Source: three-view drawing plus pictorial views. Frame: mm from the lowest corner of the part. A direction names the side the tool comes from. Coordinates: 2 decimals unless noted, no trailing zeros. Write each loop counter-clockwise with the first axis right and the second up, starting at its lowest first coordinate (ties: lowest second). Pieces come first, ordered by that corner, then holes. Notation, with made-up numbers: (40.25, -10) -> (91.25, -10) arc R22 cw to (91.25, 9) -> close; hole circle Ø4 at (10.25, 17). An arc over 180 degrees is marked (long way). One line per item, written item: value. Start each with the question number.
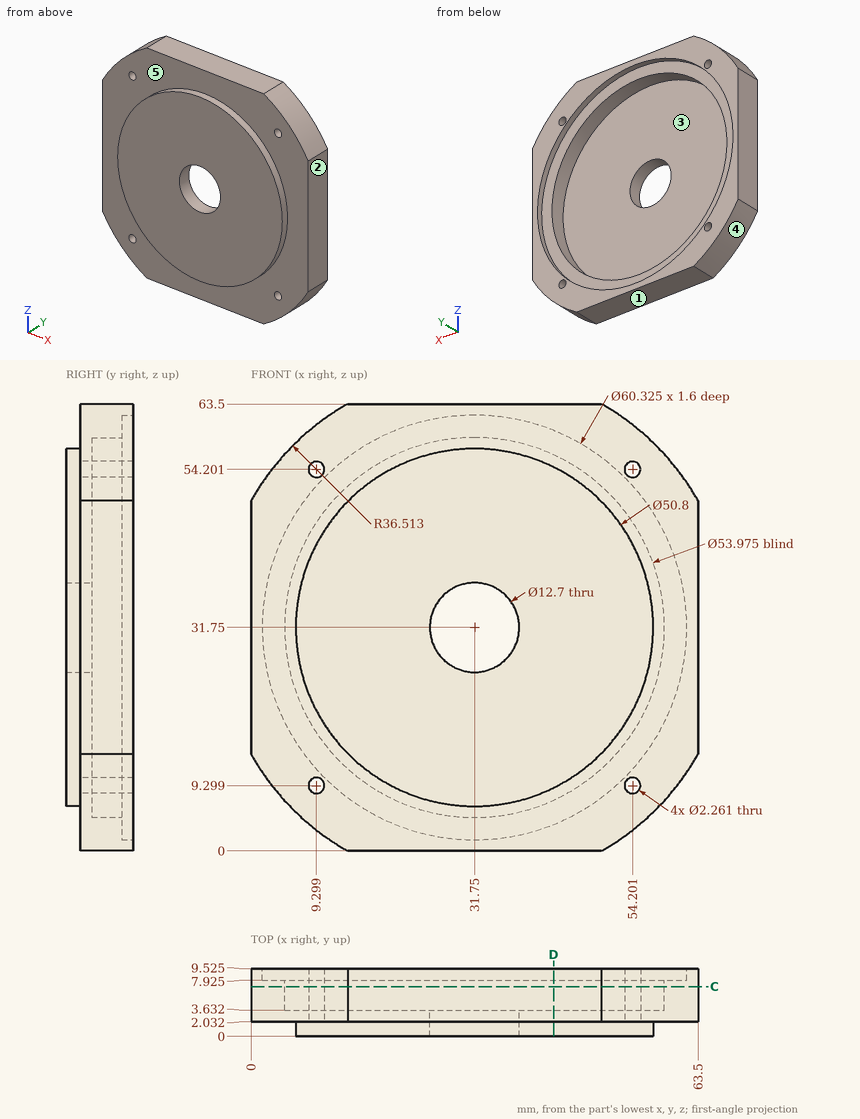
Q1. Draft query along Z for the marked faces 1, 2 and 3. Return one class per face: pulls with the +Z half, pulls with the -Z half, needs draft (parallel to the pull), parting line crosses it, or undercut.
Q2. First-contact query: P1, Ø12, axis at x = 47, z = 28.5, coming from the +Y side; P2, Ø5, axis at y = 1.5, z = 26.5, coming from the -X side; P3, Ø1.5, axis at x = 33.5, y = 1, coming from the +Z side. Flat tips, straight axial feed; report the tip coordinate or a pass-through.
Q3. Cut plane C-C on y = 7. Count the separate pieces of the cut face and the enclosed holes in it, and give its area (3 significant figures).
Q4. Access query for the marked faces 4 and 5. Directions: +Z, -Z, +X, -X, +Y, -Y. A direction counts if a zero-diameter tool reaches every point of the face in a straight line with its end or side. Return the directions, or none.
Q5. Line query: L1, parallel to Z at x = 31.75, y = 8.6; L2, parallel to X at y = 3, z = 54.5; L3, parallel to Y at x = 40.5, z = 27. Output: solid intervals per line, ascending. Write a range as from..to.
Q6. Cut plane D-D on x = 43. Output: boundary loops of the cut face in (y, z) (1 decimal).
Solution:
1. face 1: pulls with the -Z half
1. face 2: needs draft
1. face 3: undercut
2. P1: y = 3.63
2. P2: x = 0
2. P3: z = 57.13
3. separate pieces: 1
3. enclosed holes: 5
3. area: 1,420 mm²
4. face 4: -Z, -X, +Y, -Y
4. face 5: -Y
5. L1: 0..1.59, 61.91..63.5
5. L2: 3.19..8.21, 10.39..53.11, 55.29..60.31
5. L3: 0..3.63
6. outline: (0, 9) -> (2, 9) -> (2, 0) -> (9.5, 0) -> (9.5, 3.8) -> (7.9, 3.8) -> (7.9, 7.2) -> (3.6, 7.2) -> (3.6, 56.3) -> (7.9, 56.3) -> (7.9, 59.7) -> (9.5, 59.7) -> (9.5, 63.5) -> (2, 63.5) -> (2, 54.5) -> (0, 54.5) -> close
